Read the model definition and answer for the solid it produces. Units are mm, in the model's axes. Round coordinates to 2 decimals unless told otherwise and drop trailing zeros. Order: outer loops, then holes, each group sorted by start corner. A loop starts at its lowest first (then second) coordinate and runs counter-clockwise, first axis right, second up. Notation, with made-up numbers: (34, 55) - (61, 55) arc R27 cw to (61, 91) - close; hole circle Ø10 at (45.5, 69). An arc over 180 degrees is marked (long way). Answer as a JSON object with one key per item and string values. Group by question number.
Q1. A cutting plane is placed at D-D on x = 7.75. Determine the outline of the cut face in (y, z).
Q2. Given pin 1 Ø12 at (x, z) = (-8.5, 48) entering from -Y; pin 2 Ø1 at (x, z) = (3.5, 68.5) entering from -Y; pin 3 Ø12 at (y, z) = (-9.5, 60.5) entering from -X, each flat-ended and moving along its own axis, determine where each tip first touches the part or whether it passes through.
Q3. The mould has two halves that part along X. Classify faces 1 (the flat face through (-3.2, 9.2, 0)), 2 (the cylindrical face through (0.22, -19.267, 43.095)), 3 (the cylindrical face through (0.164, -17.601, 41.826)): pulls with the +X half, pulls with the -X half, needs draft (parallel to the pull), parting line crosses it, or undercut.
Q4. A cutting plane is placed at A-A on x = 0. Determine the outline of the cut face in (y, z) (3 decimals).
Q5. A cutting plane is placed at B-B on y = 0. Determine the outline of the cut face in (x, z) (3 decimals), and give its area (3 significant figures).
Q6. Consider line 1 (X direction, y = -22, z = 38.1); line 2 (Z direction, x = 0, y = -18.5); line 3 (Y direction, x = 0, z = 51.5) (3 decimals). Determine where each line is inside the solid, lowest interval first.
```python
from build123d import *

# Parameters (mm, degrees)
SWEEP1_PROFILE_R         = 13.49375
CUT_SWEEP1_PROFILE_R     = 9.525
BOSS_EXTRUDE2_DEPTH      = 12.7
BOSS_EXTRUDE2_DEPTH_BACK = 2.54
SKETCH2_R                = 5
CUT_EXTRUDE1_REACH       = 88.969
CUT_EXTRUDE1_END_RADIUS  = 9.525
SKETCH3_R                = 3.73


with BuildPart() as part:
    # Sweep1: sweep along a curve in space
    with BuildLine() as sweep1_path:
        Line((0, 0, 0), (0, 0, 76.2))
    # Sweep1 profile (on start of the path) → Sweep1 (sweep)
    with BuildSketch(Plane.XY):
        Circle(SWEEP1_PROFILE_R)
    sweep(path=sweep1_path.line)

    # Cut-Sweep1: sweep along a curve in space
    with BuildLine() as cut_sweep1_path:
        Line((0, 0, 0), (0, 0, 76.2))
    # Cut-Sweep1 profile (on start of the path) → Cut-Sweep1 (sweep, cut)
    with BuildSketch(Plane.XY):
        Circle(CUT_SWEEP1_PROFILE_R)
    sweep(path=cut_sweep1_path.line, mode=Mode.SUBTRACT)

    # Sketch2 → Boss-Extrude2 (add, two sides: drawn at the far end of the back side and taken through both)
    with BuildSketch(Plane(origin=(0, -13.49375, 0), x_dir=(-1, 0, 0), z_dir=(0, -1, 0)).offset(-BOSS_EXTRUDE2_DEPTH_BACK)):
        with Locations(Location((0, -38.1, 0), (0, 0, 90))):
            Circle(SKETCH2_R)
    extrude(amount=BOSS_EXTRUDE2_DEPTH + BOSS_EXTRUDE2_DEPTH_BACK)

    # Cut-Extrude1: up to this cylinder (the profile starts outside it)
    cut_extrude1_end = Plane(origin=(0, 0, 38.1), z_dir=(0, 0, 1)) * Cylinder(CUT_EXTRUDE1_END_RADIUS, 197.988, mode=Mode.PRIVATE)
    # Sketch3 → Cut-Extrude1 (cut, up to the surface)
    with BuildSketch(Plane.XZ.offset(26.19375), mode=Mode.PRIVATE) as cut_extrude1_sk1:
        with Locations(Location((0, 38.1, 0), (0, 0, 270))):
            Circle(SKETCH3_R)
    cut_extrude1_tool1 = extrude(cut_extrude1_sk1.sketch, amount=-CUT_EXTRUDE1_REACH, mode=Mode.PRIVATE) - cut_extrude1_end
    add(cut_extrude1_tool1.solids().sort_by_distance((0, -26.19375, 38.1))[0], mode=Mode.SUBTRACT)


solid = part.part
```
Result set:
{
 "1": {"outline": "(-11.05, 0) - (-5.54, 0) - (-5.54, 76.2) - (-11.05, 76.2) - close; (5.54, 0) - (11.05, 0) - (11.05, 76.2) - (5.54, 76.2) - close"},
 "2": {"pin 1": "stops at y = -13.26", "pin 2": "stops at y = -13.16", "pin 3": "stops at x = -13.03"},
 "3": {"face 1": "needs draft", "face 2": "parting line crosses it", "face 3": "undercut"},
 "4": {"outline": "(-26.194, 33.1) - (-13.494, 33.1) - (-13.494, 0) - (-9.525, 0) - (-9.525, 34.37) - (-26.194, 34.37) - close; (-26.194, 41.83) - (-9.525, 41.83) - (-9.525, 76.2) - (-13.494, 76.2) - (-13.494, 43.1) - (-26.194, 43.1) - close; (9.525, 0) - (13.494, 0) - (13.494, 76.2) - (9.525, 76.2) - close"},
 "5": {"outline": "(-13.494, 0) - (-9.525, 0) - (-9.525, 76.2) - (-13.494, 76.2) - close; (9.525, 0) - (13.494, 0) - (13.494, 76.2) - (9.525, 76.2) - close", "area": "605 mm²"},
 "6": {"line 1": "x = -5 to -3.73, 3.73 to 5", "line 2": "z = 33.1 to 34.37, 41.83 to 43.1", "line 3": "y = -13.494 to -9.525, 9.525 to 13.494"}
}
